from build123d import *

# Parameters (mm, degrees)
BOSS_EXTRUDE1_DEPTH      = 2
BOSS_EXTRUDE3_DEPTH      = 1
BOSS_EXTRUDE3_DEPTH_BACK = 3
SKETCH3_W                = 5
SKETCH3_H                = 4
SKETCH3_R                = 1.980106187
CUT_EXTRUDE1_DEPTH       = 7.545644
CUT_EXTRUDE2_DEPTH       = 8
SKETCH6_R                = 0.4
CUT_EXTRUDE3_DEPTH       = 4


with BuildPart() as part:
    # Sketch1 → Boss-Extrude1 (new body)
    with BuildSketch(Plane.XY):
        with BuildLine():
            ThreePointArc((0, 2), (1.414213562, 1.414213562), (2, 0))
            Line((2, 0), (6, 0))
            ThreePointArc((6, 0), (0, 6), (-6, 0))
            Line((-6, 0), (-2, 0))
            ThreePointArc((-2, 0), (-1.414213562, 1.414213562), (0, 2))
        make_face()
        with BuildLine():
            Line((6, 0), (2, 0))
            ThreePointArc((2, 0), (1.414213562, -1.414213562), (0, -2))
            ThreePointArc((0, -2), (-1.414213562, -1.414213562), (-2, 0))
            Line((-2, 0), (-6, 0))
            ThreePointArc((-6, 0), (0, -6), (6, 0))
        make_face()
    extrude(amount=-BOSS_EXTRUDE1_DEPTH)

    # Sketch2 → Boss-Extrude3 (add, two sides: drawn at the far end of the back side and taken through both)
    with BuildSketch(Plane.XY.offset(-BOSS_EXTRUDE3_DEPTH_BACK)):
        Polygon((-2.5, -13), (2.5, -13), (2.5, -5.454356057), (2.5, -2), (-2.5, -2), (-2.5, -5.454356057), align=None)
    extrude(amount=BOSS_EXTRUDE3_DEPTH + BOSS_EXTRUDE3_DEPTH_BACK)

    # Sketch3 → Cut-Extrude1 (cut)
    with BuildSketch(Plane.XZ.offset(13)):
        with Locations((0, -1)):
            Rectangle(SKETCH3_W, SKETCH3_H)
        with Locations((0, -1)):
            Circle(SKETCH3_R, mode=Mode.SUBTRACT)
    extrude(amount=-CUT_EXTRUDE1_DEPTH, mode=Mode.SUBTRACT)

    # Sketch5 → Cut-Extrude2 (cut)
    with BuildSketch(Plane(origin=(2.5, 0, 0), x_dir=(0, 0, -1), z_dir=(1, 0, 0))):
        Polygon((-1, -5.454356057), (0, -2), (-1, -2), align=None)
        Polygon((3, -5.454356057), (2, -2), (3, -2), align=None)
    extrude(amount=-CUT_EXTRUDE2_DEPTH, mode=Mode.SUBTRACT)

    # Sketch6 → Cut-Extrude3 (cut)
    with BuildSketch(Plane.XZ.offset(13)):
        with Locations((0, -1)):
            Circle(SKETCH6_R)
    extrude(amount=-CUT_EXTRUDE3_DEPTH, mode=Mode.SUBTRACT)


solid = part.part
Check sheet for the modelled part. Datum: model origin and axes. Units: mm. A direction names the side the tool comes from. Give positions to 0.01 mm unless a question says otherwise; leave off trailing zeros. Loops run counter-clockwise (first coordinate to the right, second up) from the corner with the lowest first, then second, coordinate; pieces in that order, holes last. Notation, with made-up numbers: M 8.25,-26.5 L 53.25,-26.5 A28 cw 53.25,1.5 Z; hole C 19,71 d1. An arc over 180 degrees is marked long. Use a Markdown table: item, result. Add a question column.
Q1. Tool access check on faces 1 (the flat face through (-2.5, -4.5, 0.3)), 2 (the flat face through (2.5, -4.1, 0.4)), 3 (the flat face through (1, 2, -2)), 4 (the flat face through (2.5, -4.5, -2.3)), 5 (the cylindrical face through (-1.571, -9.28, -2.205)). Record the directions out of +Z, -Z, +X, -X, +Y, -Y that give a thin tool (end or side, any length) a straight path to the whole face; none if there is none.
Q2. Sectioned sample at B-B, the plane y = -4.5. Record the cut outline in (x, z), then the cut area to 3 significant figures.
Q3. Scan lines: line 1 along Z through (x, y) = (0, -10.85); line 2 along Y through (x, z) = (1.75, -1.8); line 3 along Z through (x, y) = (-2.75, -2.5). Record each from-to range of solid material in increasing order. Write a range as [from, to].
Q4. Sectioned sample at C-C, the plane z = -2.3. Record the cut outline in (x, y).
Q5. Go/stop test with flat-tipped pins: pin 1 (0.6 mm diameter, centred on x = 0, z = -1, fed in from -Y); pin 2 (6 mm diameter, centred on x = 3.5, y = 1, fed in from +Z); pin 3 (4 mm diameter, centred on x = -3, y = -9.5, fed in from +Z); pin 4 (1.5 mm diameter, centred on x = 4.5, y = -9, fed in from +Z). Record where each tip stops, or that it passes through.
Q6. Sectioned sample at D-D, the plane x = -4.5. Record the cut outline in (y, z), then the cut area to 3 significant figures.
Q7. Sectioned sample at A-A, the plane z = -1. Record the cut outline in (x, y).
Verdict:
| question | item | result |
|---|---|---|
| 1 | face 1 | +Z, -X, +Y, -Y |
| 1 | face 2 | +Z, +X, +Y, -Y |
| 1 | face 3 | -Z, +Y |
| 1 | face 4 | -Z, +X, +Y, -Y |
| 1 | face 5 | -Y |
| 2 | outline | M -3.97,-2 L -2.5,-2 L -2.5,-2.72 L 2.5,-2.72 L 2.5,-2 L 3.97,-2 L 3.97,0 L 2.5,0 L 2.5,0.72 L -2.5,0.72 L -2.5,0 L -3.97,0 Z |
| 2 | area | 23.1 mm^2 |
| 3 | line 1 | [-2.98, -1.4], [-0.6, 0.98] |
| 3 | line 2 | [-13, -0.97], [0.97, 5.74] |
| 3 | line 3 | [-2, 0] |
| 4 | outline | M -2.5,-5.45 L -1.49,-5.45 L -1.49,-13 L 1.49,-13 L 1.49,-5.45 L 2.5,-5.45 L 2.5,-3.04 L -2.5,-3.04 Z |
| 5 | pin 1 | y = -9 |
| 5 | pin 2 | z = 0 |
| 5 | pin 3 | z = 0.71 |
| 5 | pin 4 | through |
| 6 | outline | M -3.97,-2 L 3.97,-2 L 3.97,0 L -3.97,0 Z |
| 6 | area | 15.9 mm^2 |
| 7 | outline | M -2.5,-5.45 L -1.98,-5.45 L -1.98,-13 L -0.4,-13 L -0.4,-9 L 0.4,-9 L 0.4,-13 L 1.98,-13 L 1.98,-5.45 L 2.5,-5.45 A6 ccw long Z; hole C 0,0 d4 |
